Check sheet for the modelled part. Datum: model origin and axes. Units: mm. Face numbers are marked on the shaded views. Round coordinates to 2 decimals unless told otherwise and drop trailing zeros. Loops run counter-clockwise (first coordinate to the right, second up) from the corner with the lowest first, then second, coordinate; pieces in that order, holes last. Notation, with made-up numbers: (24, 25.25) - (38, 25.25) arc R24 cw to (38, 62.25) - close; hole circle Ø2 at (52.5, 46). An arc over 180 degrees is marked (long way). Answer in a Markdown table with one row per item. Add a question column.
(1) Mould release check, pull along Z, two halves, no side actions. Record for the marked faces 1, 2 and 3: +Z half, -Z half, draft (parallel to the pull), parting line (faces both ways), or undercut.
(2) Cross-section at B-B on z = 8.25. Enter the section's corners in (x, y) (3 decimals), then the cut area to 3 significant figures.
(3) Cross-section at A-A on y = 0. Enter the section's corners in (x, z) (3 decimals).
(4) Cross-section at C-C on x = 4.75. Enter the section's corners in (y, z) (3 decimals).
(5) Thickness scan on line 1 along Y through (x, z) = (1.75, 6.25); line 2 along Z through (x, y) = (-4.5, 0) (3 decimals); line 3 along X through (y, z) = (0, 11) (3 decimals). Record the ranges inside material, lowest first.
(6) Cross-section at D-D on z = 10.25. Enter the section's corners in (x, y) (3 decimals), then the cut area to 3 significant figures.
Autodesk Inventor part; units mm, degrees
ref_plane "YZ Plane" through (0, 0, 0) normal (1, 0, 0) x (0, 1, 0)
ref_plane "XZ Plane" through (0, 0, 0) normal (0, 1, 0) x (-1, 0, 0)
ref_plane "XY Plane" through (0, 0, 0) normal (0, 0, 1) x (1, 0, 0)
sketch "Sketch1" plane through (0, 0, 0) normal (0, 0, 1) x (1, 0, 0)
  line L0 (-6.35, 6.35) -> (6.35, 6.35)
  line L1 (6.35, 6.35) -> (6.35, -6.35)
  line L2 (6.35, -6.35) -> (-6.35, -6.35)
  line L3 (-6.35, -6.35) -> (-6.35, 6.35)
  line L4 (-6.35, 6.35) -> (6.35, -6.35) construction
  line L5 (6.35, 6.35) -> (-6.35, -6.35) construction
  point P0 (0, 0)
  dimension "d0" = 12.7
  dimension "d1" = 12.7
extrude "Extrusion1" add sketch "Sketch1" along normal blind 12.7
sketch "Sketch4" plane through (0, 0, 12.7) normal (0, 0, 1) x (1, 0, 0)
  point P0 (0, 0)
hole "Hole1" at (0, 0, 12.7) direction (0, 0, -1) diameter 6.35 end through all
sketch "Sketch5" plane through (6.35, -6.35, 0) normal (1, 0, 0) x (0, 0, -1)
  line L0 (-12.7, 12.7) -> (0, 0)
  point P0 (0, 6.35)
  point P1 (-6.35, 6.35)
hole "Hole2" at (6.35, 0, 6.35) direction (-1, 0, 0) diameter 6.35 end through all
equation "\"d0\" = d1"
properties part number "Connector" material "Nylon 6/6"
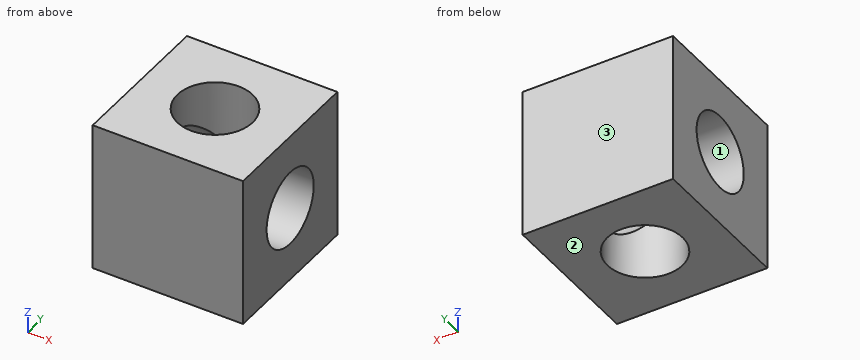
Answers:
| question | item | result |
|---|---|---|
| 1 | face 1 | undercut |
| 1 | face 2 | -Z half |
| 1 | face 3 | draft |
| 2 | outline | (-6.35, -6.35) - (6.35, -6.35) - (6.35, -2.544) - (1.9, -2.544) arc R3.175 cw to (-1.9, -2.544) - (-6.35, -2.544) - close; (-6.35, 2.544) - (-1.9, 2.544) arc R3.175 cw to (1.9, 2.544) - (6.35, 2.544) - (6.35, 6.35) - (-6.35, 6.35) - close |
| 2 | area | 93.4 mm^2 |
| 3 | outline | (-6.35, 0) - (-3.175, 0) - (-3.175, 3.175) - (-6.35, 3.175) - close; (-6.35, 9.525) - (-3.175, 9.525) - (-3.175, 12.7) - (-6.35, 12.7) - close; (3.175, 0) - (6.35, 0) - (6.35, 3.175) - (3.175, 3.175) - close; (3.175, 9.525) - (6.35, 9.525) - (6.35, 12.7) - (3.175, 12.7) - close |
| 4 | outline | (-6.35, 0) - (6.35, 0) - (6.35, 12.7) - (-6.35, 12.7) - close; hole circle Ø6.35 at (0, 6.35) |
| 5 | line 1 | y = -6.35 to -3.17, 3.17 to 6.35 |
| 5 | line 2 | z = 0 to 3.175, 9.525 to 12.7 |
| 5 | line 3 | x = -6.35 to -3.175, 3.175 to 6.35 |
| 6 | outline | (-6.35, -6.35) - (6.35, -6.35) - (6.35, 6.35) - (-6.35, 6.35) - close; hole circle Ø6.35 at (0, 0) |
| 6 | area | 130 mm^2 |
